```python
from build123d import *

# Parameters (mm, degrees)
BOSS_EXTRUDE1_DEPTH = 3.048


with BuildPart() as part:
    # Sketch1 → Boss-Extrude1 (new body)
    with BuildSketch(Plane.XY):
        Polygon((-22.225, -3.048), (-19.558, -3.048), (-19.558, 0), (-5.715, 0), (-5.715, -3.048), (-3.175, -3.048), (-3.175, -13.335), (0, -13.335), (0, -48.895), (-3.175, -48.895), (-3.175, -59.182), (-5.715, -59.182), (-5.715, -62.23), (-19.558, -62.23), (-19.558, -59.182), (-22.225, -59.182), (-22.225, -52.832), (-25.273, -52.832), (-25.273, -41.402), (-22.225, -41.402), (-22.225, -20.828), (-25.273, -20.828), (-25.273, -9.398), (-22.225, -9.398), align=None)
    extrude(amount=BOSS_EXTRUDE1_DEPTH)


solid = part.part
```
The listing builds one solid part. Answer for the finished solid, in the listing's coordinates (mm). A direction names the side the tool comes from. Coordinates: 2 decimals unless noted, no trailing zeros. Order: outer loops, then holes, each group sorted by start corner. A loop starts at its lowest first (then second) coordinate and runs counter-clockwise, first axis right, second up. Notation, with made-up numbers: M 23.5,5.5 L 63.5,5.5 A18 cw 63.5,10.5 Z; hole C 57.25,14 d6. An arc over 180 degrees is marked long. Answer as a JSON object with one key per item and string values. Group by question number.
1. Section D-D on y = -34 is taken. Write down the section's boundary in (x, z) (3 decimals), then the cut area to 3 significant figures.
2. Flat-ended cylindrical pins translate along their axes: P1, Ø1.5, axis at y = -61, z = 1.5, coming from the +X side (3 decimals); P2, Ø1.5, axis at y = -54.5, z = 1.5, coming from the -X side (3 decimals); P3, Ø0.9, axis at y = -60.5, z = 1.5, coming from the -X side. Find the tip coordinate at first contact, or state that the pin passes through.
3. Section B-B on z = 1.9 is taken. Write down the section's boundary in (x, y) (3 decimals).
4. A tool of negligible diameter and unlimited length cuts with its end or side. For faces 1 (the flat face through (-19.558, -2, 2)), 2 (the flat face through (-2, -13.335, 2)), 3 (the flat face through (-24, -20.828, 2)), from which of +Z, -Z, +X, -X, +Y, -Y can it reach the whole face along a straight path? Write none if from no direction.
5. Section A-A on x = -23 is taken. Write down the section's boundary in (y, z).
6. Straight lines are drawn through the part: line 1 (Y direction, x = -23, z = 2.95); line 2 (X direction, y = -38, z = 2) (3 decimals); line 3 (Y direction, x = -3.5, z = 2.4). For each, find the intervals that lie inside material, in ascending order.
7. Section C-C on x = -1.5 is taken. Write down the section's boundary in (y, z) (3 decimals).
Values follow:
{
 "1": {"outline": "M -22.225,0 L 0,0 L 0,3.048 L -22.225,3.048 Z", "area": "67.7 mm2"},
 "2": {"P1": "x = -5.715", "P2": "x = -22.225", "P3": "x = -19.56"},
 "3": {"outline": "M -25.273,-52.832 L -22.225,-52.832 L -22.225,-59.182 L -19.558,-59.182 L -19.558,-62.23 L -5.715,-62.23 L -5.715,-59.182 L -3.175,-59.182 L -3.175,-48.895 L 0,-48.895 L 0,-13.335 L -3.175,-13.335 L -3.175,-3.048 L -5.715,-3.048 L -5.715,0 L -19.558,0 L -19.558,-3.048 L -22.225,-3.048 L -22.225,-9.398 L -25.273,-9.398 L -25.273,-20.828 L -22.225,-20.828 L -22.225,-41.402 L -25.273,-41.402 Z"},
 "4": {"face 1": "+Z, -Z, -X, +Y", "face 2": "+Z, -Z, +X, +Y", "face 3": "+Z, -Z, -X"},
 "5": {"outline": "M -52.83,0 L -41.4,0 L -41.4,3.05 L -52.83,3.05 Z; M -20.83,0 L -9.4,0 L -9.4,3.05 L -20.83,3.05 Z"},
 "6": {"line 1": "-52.83 to -41.4, -20.83 to -9.4", "line 2": "-22.225 to 0", "line 3": "-59.18 to -3.05"},
 "7": {"outline": "M -48.895,0 L -13.335,0 L -13.335,3.048 L -48.895,3.048 Z"}
}
